Here's how the part is built. I have some questions about the finished solid (model axes, mm). Give positions to 0.01 mm unless a question says otherwise; leave off trailing zeros. Loops run counter-clockwise (first coordinate to the right, second up) from the corner with the lowest first, then second, coordinate; pieces in that order, holes last.
Q1. I'm going to push a flat-ended pin straight in: P1, Ø1.9, axis at x = 0, z = 0, coming from the +Y side. Where does the tip first touch, or does it pass through?
Q2. Suppose I cut it at C-C (y = 3.2). List the corners of the cut face in (x, z) for me, and give its area (3 significant figures).
Q3. I need wall thicknesses on probe 1 along Z at (x, y) = (0, 0.9); probe 2 along X at (y, z) = (3.4, -0.5). Which ranges of each line are inside material? Lowest first, please.
Q4. Suppose I cut it at B-B (x = 1). List the corners of the cut face in (y, z) for me, and give its area (3 significant figures).
Q5. Thinking about a two-plate mould opening in Z: for faces 1 (the face through (-1, 0, 2)), 2 (the face through (1.081, 2.169, 3.434)), 3 (the face through (0.481, 2.169, 1.526)), which applies, pulls with the +Z half, pulls with the -Z half, needs draft (parallel to the pull), parting line crosses it, or undercut?
Q6. Suppose I cut it at D-D (z = -0.75). List the corners of the cut face in (x, y) for me, and give its area (3 significant figures).
```python
from build123d import *

# Parameters (mm, degrees)
SKETCH_1_R               = 3.6
SKETCH_1_R_2             = 1.6
EXTRUDE_1_DEPTH          = 4.4
CUT_EXTRUDE_1_DEPTH      = 10
CUT_EXTRUDE_1_DEPTH_BACK = 10


with BuildPart() as part:
    # Sketch 1 → Extrude 1 (new body)
    with BuildSketch(Plane(origin=(0, 0, 0), x_dir=(1, 0, 0), z_dir=(0, 1, 0))):
        with Locations(Location((0, 0, 0), (0, 0, 270))):
            Circle(SKETCH_1_R)
        with Locations(Location((0, 0, 0), (0, 0, 270))):
            Circle(SKETCH_1_R_2, mode=Mode.SUBTRACT)
    extrude(amount=EXTRUDE_1_DEPTH)

    # Sketch 2 → Cut-Extrude 1 (cut, two sides: drawn at the far end of the back side and taken through both)
    with BuildSketch(Plane.XY.offset(-CUT_EXTRUDE_1_DEPTH_BACK)):
        Polygon((-2.8, 4.4), (-3.6, 4.4), (-3.2, 4), align=None)
        Polygon((3.6, 4.4), (2.8, 4.4), (3.2, 4), align=None)
        Polygon((2.8, 4.4), (2, 4.4), (2.4, 4), align=None)
        Polygon((2, 4.4), (1.2, 4.4), (1.6, 4), align=None)
        Polygon((1.2, 4.4), (0.4, 4.4), (0.8, 4), align=None)
        Polygon((0.4, 4.4), (-0.4, 4.4), (0, 4), align=None)
        Polygon((-0.4, 4.4), (-1.2, 4.4), (-0.8, 4), align=None)
        Polygon((-1.2, 4.4), (-2, 4.4), (-1.6, 4), align=None)
        Polygon((-2, 4.4), (-2.8, 4.4), (-2.4, 4), align=None)
    extrude(amount=CUT_EXTRUDE_1_DEPTH + CUT_EXTRUDE_1_DEPTH_BACK, mode=Mode.SUBTRACT)


solid = part.part
```
Solutions:
1. P1: passes through
2. outline: circle Ø7.2 at (0, 0); hole circle Ø3.2 at (0, 0)
2. area: 32.7 mm2
3. probe 1: z = -3.6 to -1.6, 1.6 to 3.6
3. probe 2: x = -3.57 to -1.52, 1.52 to 3.57
4. outline: (0, -3.46) - (4.2, -3.46) - (4.2, -1.25) - (0, -1.25) - close; (0, 1.25) - (4.2, 1.25) - (4.2, 3.46) - (0, 3.46) - close
4. area: 18.6 mm2
5. face 1: needs draft
5. face 2: parting line crosses it
5. face 3: undercut
6. outline: (-3.52, 0) - (-1.41, 0) - (-1.41, 4.19) - (-1.6, 4) - (-2, 4.4) - (-2.4, 4) - (-2.8, 4.4) - (-3.2, 4) - (-3.52, 4.32) - close; (1.41, 0) - (3.52, 0) - (3.52, 4.32) - (3.2, 4) - (2.8, 4.4) - (2.4, 4) - (2, 4.4) - (1.6, 4) - (1.41, 4.19) - close
6. area: 17.6 mm2
